For this review, take the finished solid that the model builds, in its own axes (mm). A direction names the side the tool comes from. Give positions to 0.01 mm unless a question says otherwise; leave off trailing zeros. Write each loop counter-clockwise with the first axis right and the second up, starting at its lowest first coordinate (ties: lowest second). Pieces come first, ordered by that corner, then holes. Notation, with made-up numbers: (30, -10) -> (82, -10) arc R37 cw to (82, 28) -> close; hole circle Ø5 at (-38.75, 24). An arc over 180 degrees is marked (long way). Return JSON: item names as keys, results as strings.
from build123d import *

# Parameters (mm, degrees)
SKETCH1_W            = 68.248659994
SKETCH1_H            = 70.504814042
BOSS_EXTRUDE1_DEPTH  = 2.54
M5_CLEARANCE_HOLE1_D = 5.5
CUT_EXTRUDE1_DEPTH   = 50.128949699


with BuildPart() as part:
    # Sketch1 → Boss-Extrude1 (new body)
    with BuildSketch(Plane(origin=(0, 0, 0), x_dir=(1, 0, 0), z_dir=(0, 1, 0))):
        Rectangle(SKETCH1_W, SKETCH1_H)
    extrude(amount=BOSS_EXTRUDE1_DEPTH)

    # M5 Clearance Hole1 (through all)
    with Locations(Plane(origin=(0, 2.54, 0), x_dir=(1, 0, 0), z_dir=(0, 1, 0))):
        with Locations((26, 27), (-26, 27), (-26, -27), (26, -27)):
            Hole(M5_CLEARANCE_HOLE1_D / 2)

    # Sketch2 → Cut-Extrude1 (cut, through all)
    with BuildSketch(Plane(origin=(0, 2.54, 0), x_dir=(1, 0, 0), z_dir=(0, 1, 0))):
        with BuildLine():
            Line((-4.75, 14.7), (4.75, 14.7))
            Line((4.75, 14.7), (4.75, 9.310612225))
            ThreePointArc((4.75, 9.310612225), (22.581133525, -3.075464159), (0.916994756, -4.5))
            Line((0.916994756, -4.5), (-0.916994756, -4.5))
            ThreePointArc((-0.916994756, -4.5), (-22.581133525, -3.075464159), (-4.75, 9.310612225))
            Line((-4.75, 9.310612225), (-4.75, 14.7))
        make_face()
    extrude(amount=-CUT_EXTRUDE1_DEPTH, mode=Mode.SUBTRACT)


solid = part.part
1. To check wall thickness, follow probe 1 along Z at (x, y) = (26, 1.3); probe 2 along X at (y, z) = (0.7, 27); probe 3 along X at (y, z) = (1.6, 0). State the ranges of each line that lie inside material, in increasing order.
Results found:
{"probe 1": "z = -35.25 to -29.75, -24.25 to 24.25, 29.75 to 35.25", "probe 2": "x = -34.12 to -28.75, -23.25 to 23.25, 28.75 to 34.12", "probe 3": "x = -34.12 to -23, 23 to 34.12"}
2. The part is to be moulded in two halves that separate along X. For faces 3 (the flat face through (34.124, 1, 0)), 4 (the flat face through (0, 1, 4.5)), 5 (the flat face through (0, 0, 7)), say which applies: +X half, -X half, draft (parallel to the pull), parting line (faces both ways), or undercut.
Results found:
{"face 3": "+X half", "face 4": "undercut", "face 5": "draft"}
3. Add section D-D, the plane x = -26. State the section outline as (y, z) points, plus the area to 3 significant figures.
Results found:
{"outline": "(0, -35.25) -> (2.54, -35.25) -> (2.54, -29.75) -> (0, -29.75) -> close; (0, -24.25) -> (2.54, -24.25) -> (2.54, 24.25) -> (0, 24.25) -> close; (0, 29.75) -> (2.54, 29.75) -> (2.54, 35.25) -> (0, 35.25) -> close", "area": "151 mm²"}
4. Add section C-C, the plane y = 0.5. State the section outline as (x, z) points.
Results found:
{"outline": "(-34.12, -35.25) -> (34.12, -35.25) -> (34.12, 35.25) -> (-34.12, 35.25) -> close; hole circle Ø5.5 at (-26, -27); hole circle Ø5.5 at (-26, 27); hole (-4.75, -14.7) -> (4.75, -14.7) -> (4.75, -9.31) arc R11.5 ccw (long way) to (0.92, 4.5) -> (-0.92, 4.5) arc R11.5 ccw (long way) to (-4.75, -9.31) -> close; hole circle Ø5.5 at (26, -27); hole circle Ø5.5 at (26, 27)"}
5. Add section A-A, the plane x = 11.5. State the section outline as (y, z) points.
Results found:
{"outline": "(0, -35.25) -> (2.54, -35.25) -> (2.54, -11.5) -> (0, -11.5) -> close; (0, 11.5) -> (2.54, 11.5) -> (2.54, 35.25) -> (0, 35.25) -> close"}
6. For faces 1 (the flat face through (0, 1, -35.252)), 2 (the flat face through (4.75, 1, -12)), list the 3-axis set-ups (+Z, -Z, +X, -X, +Y, -Y) from which the entire face can be reached by the end or side of a thin tool; tool diameter is ignored.
Results found:
{"face 1": "-Z, +X, -X, +Y, -Y", "face 2": "+Y, -Y"}
7. Add section B-B, the plane z = 27. State the section outline as (x, y) points, plus the area to 3 significant figures.
Results found:
{"outline": "(-34.12, 0) -> (-28.75, 0) -> (-28.75, 2.54) -> (-34.12, 2.54) -> close; (-23.25, 0) -> (23.25, 0) -> (23.25, 2.54) -> (-23.25, 2.54) -> close; (28.75, 0) -> (34.12, 0) -> (34.12, 2.54) -> (28.75, 2.54) -> close", "area": "145 mm²"}
